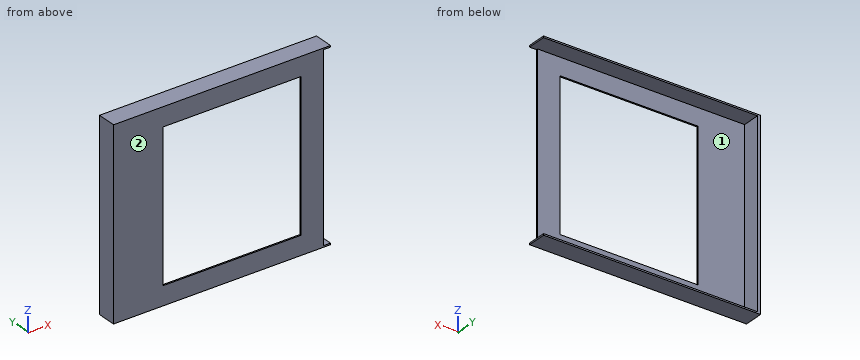
from build123d import *

# Parameters (mm, degrees)
F0_W     = 138
F0_H     = 121
F0_W_2   = 92
F0_H_2   = 98
F1_DEPTH = 12.8
F2_DEPTH = 11.8
F3_DEPTH = 12.8
F0_W_3   = 4.8031793237
F0_H_3   = 1
F0_W_4   = 4.8
F4_DEPTH = 12.8


with BuildPart() as f1:
    # F0 (on Front) → F1 (new body)
    with BuildSketch(Plane.XZ):
        with Locations((-3.5, 0)):
            Rectangle(F0_W, F0_H)
        with Locations((4.5, 0)):
            Rectangle(F0_W_2, F0_H_2, mode=Mode.SUBTRACT)
        with Locations((4.5, 0)):
            Rectangle(F0_W_2, F0_H_2)
        Polygon((-74.5, 61.5), (-74.5, -61.5), (65.5, -61.5), (65.5, -60.5), (-72.5, -60.5), (-72.5, 60.5), (65.5, 60.5), (65.5, 61.5), align=None)
    extrude(amount=F1_DEPTH)

    # F0 (on Front) → F2 (cut)
    with BuildSketch(Plane.XZ):
        with Locations((-3.5, 0)):
            Rectangle(F0_W, F0_H)
        with Locations((4.5, 0)):
            Rectangle(F0_W_2, F0_H_2, mode=Mode.SUBTRACT)
        with Locations((4.5, 0)):
            Rectangle(F0_W_2, F0_H_2)
    extrude(amount=F2_DEPTH, mode=Mode.SUBTRACT)

    # F0 (on Front) → F3 (cut)
    with BuildSketch(Plane.XZ):
        with Locations((4.5, 0)):
            Rectangle(F0_W_2, F0_H_2)
    extrude(amount=F3_DEPTH, mode=Mode.SUBTRACT)

    # F0 (on Front) → F4 (join)
    with BuildSketch(Plane.XZ):
        with Locations((67.9015896618, 61)):
            Rectangle(F0_W_3, F0_H_3)
        with Locations((67.9, -61)):
            Rectangle(F0_W_4, F0_H_3)
    extrude(amount=F4_DEPTH)


solid = f1.part
Model file for the job. Use its own axes, mm. Face numbers are marked on the shaded views. A direction names the side the tool comes from. Give positions to 0.01 mm unless a question says otherwise; leave off trailing zeros. Order: outer loops, then holes, each group sorted by start corner. A loop starts at its lowest first (then second) coordinate and runs counter-clockwise, first axis right, second up. Notation, with made-up numbers: (58.5, 75) - (84.5, 75) arc R27 cw to (84.5, 105) - close; hole circle Ø4 at (-29.5, 88.5). An arc over 180 degrees is marked (long way). One line per item, written item: value.
Item 1: Slice it at B-B (x = 15). List the corners of the cut face in (y, z).
Response values:
outline: (-12.8, -61.5) - (0, -61.5) - (0, -60.5) - (-11.8, -60.5) - (-11.8, -49) - (-12.8, -49) - close; (-12.8, 49) - (-11.8, 49) - (-11.8, 60.5) - (0, 60.5) - (0, 61.5) - (-12.8, 61.5) - close
Item 2: Wall check: line 1 (Z direction, x = -34, y = -4.75); line 2 (Z direction, x = -4.5, y = -12); line 3 (X direction, y = -5, z = 28). Give the ranges that are in metal, low to high.
Response values:
line 1: -61.5 to -60.5, 60.5 to 61.5
line 2: -61.5 to -49, 49 to 61.5
line 3: -74.5 to -72.5
Item 3: Slice it at D-D (x = -61.5). List the corners of the cut face in (y, z).
Response values:
outline: (-12.8, -61.5) - (0, -61.5) - (0, -60.5) - (-11.8, -60.5) - (-11.8, 60.5) - (0, 60.5) - (0, 61.5) - (-12.8, 61.5) - close
Item 4: Tool access for the marked faces 1 and 2: list every direction of +Z, -Z, +X, -X, +Y, -Y with a clear straight run to the whole face (end or side of a thin tool).
Response values:
face 1: +X, +Y
face 2: +Z, -Z, +X, -X, -Y
Item 5: Slice it at C-C (y = -4). List the corners of the cut face in (x, z).
Response values:
outline: (-74.5, -61.5) - (70.3, -61.5) - (70.3, -60.5) - (-72.5, -60.5) - (-72.5, 60.5) - (70.3, 60.5) - (70.3, 61.5) - (-74.5, 61.5) - close
Item 6: Pin check, flat tips, straight feed: pin 1 Ø10 at (x, z) = (-50, -21.5) entering from +Y; pin 2 Ø1.5 at (y, z) = (-5, 36) entering from +X; pin 3 Ø1.1 at (y, z) = (-12, 4) entering from +X. Stop position of each tip, or through.
Response values:
pin 1: y = -11.8
pin 2: x = -72.5
pin 3: x = 65.5
Item 7: Slice it at A-A (z = -14.5). List the corners of the cut face in (x, y).
Response values:
outline: (-74.5, -12.8) - (-41.5, -12.8) - (-41.5, -11.8) - (-72.5, -11.8) - (-72.5, 0) - (-74.5, 0) - close; (50.5, -12.8) - (65.5, -12.8) - (65.5, -11.8) - (50.5, -11.8) - close
